Input: part model. Units: mm. Frame: model coordinates. A direction names the side the tool comes from. Coordinates: 2 decimals unless noted, no trailing zeros. Loops run counter-clockwise (first coordinate to the right, second up) from the corner with the lowest first, then second, coordinate; pieces in that order, holes last.
```python
from build123d import *

# Parameters (mm, degrees)
F2_DEPTH = 0.1
F3_ANGLE = 180
F4_ANGLE = 180
F5_DEPTH = 0.1
F6_R     = 0.2427611579
F7_DEPTH = 1


with BuildPart() as f2:
    # F1 (on Front) → F2 (new body)
    with BuildSketch(Plane.XZ):
        with BuildLine():
            Line((0, 0.6), (0, 0))
            Line((0, 0), (5, 0))
            Line((5, 0), (7.4486832981, 7.3460498942))
            ThreePointArc((7.4486832981, 7.3460498942), (7.4870874576, 7.5020954172), (7.5, 7.6622776602))
            Line((7.5, 7.6622776602), (7.5, 16.6690481052))
            ThreePointArc((7.5, 16.6690481052), (7.3911447846, 17.4698488508), (7.0724787771, 18.2125353714))
            Line((7.0724787771, 18.2125353714), (3.1456512734, 24.7572478777))
            ThreePointArc((3.1456512734, 24.7572478777), (2.963254218, 24.9350999534), (2.7169048105, 25))
            Line((2.7169048105, 25), (0, 25))
            Line((0, 25), (0, 24.4))
            Line((0, 24.4), (2.6383143499, 24.4))
            ThreePointArc((2.6383143499, 24.4), (2.6777302551, 24.3896159925), (2.7069137839, 24.3611596604))
            Line((2.7069137839, 24.3611596604), (6.5751328802, 17.9141278333))
            ThreePointArc((6.5751328802, 17.9141278333), (6.8321901263, 17.3150273733), (6.92, 16.6690481052))
            Line((6.92, 16.6690481052), (6.92, 7.6622776602))
            ThreePointArc((6.92, 7.6622776602), (6.9145767322, 7.5950011181), (6.8984469852, 7.5294619984))
            Line((6.8984469852, 7.5294619984), (4.588626319, 0.6))
            Line((4.588626319, 0.6), (0, 0.6))
        make_face()
    extrude(amount=F2_DEPTH)

    # F2_face (on face) → F3 (revolve)
    with BuildSketch(Plane(origin=(5.1843610202, -0.1, 11.965116571), x_dir=(1, 0, 0), z_dir=(0, -1, 0))):
        with BuildLine():
            Line((-0.5957347012, -11.365116571), (-5.1843610202, -11.365116571))
            Line((-5.1843610202, -11.365116571), (-5.1843610202, -11.965116571))
            Line((-5.1843610202, -11.965116571), (-0.1843610202, -11.965116571))
            Line((-0.1843610202, -11.965116571), (2.2643222778, -4.6190666769))
            ThreePointArc((2.2643222778, -4.6190666769), (2.3027264374, -4.4630211539), (2.3156389798, -4.3028389109))
            Line((2.3156389798, -4.3028389109), (2.3156389798, 4.7039315341))
            ThreePointArc((2.3156389798, 4.7039315341), (2.2067837644, 5.5047322798), (1.8881177569, 6.2474188004))
            Line((1.8881177569, 6.2474188004), (-2.0387097468, 12.7921313067))
            ThreePointArc((-2.0387097468, 12.7921313067), (-2.2211068022, 12.9699833824), (-2.4674562097, 13.034883429))
            Line((-2.4674562097, 13.034883429), (-5.1843610202, 13.034883429))
            Line((-5.1843610202, 13.034883429), (-5.1843610202, 12.434883429))
            Line((-5.1843610202, 12.434883429), (-2.5460466703, 12.434883429))
            ThreePointArc((-2.5460466703, 12.434883429), (-2.5066307651, 12.4244994215), (-2.4774472363, 12.3960430894))
            Line((-2.4774472363, 12.3960430894), (1.39077186, 5.9490112623))
            ThreePointArc((1.39077186, 5.9490112623), (1.6478291061, 5.3499108023), (1.7356389798, 4.7039315341))
            Line((1.7356389798, 4.7039315341), (1.7356389798, -4.3028389109))
            ThreePointArc((1.7356389798, -4.3028389109), (1.730215712, -4.3701154529), (1.714085965, -4.4356545726))
            Line((1.714085965, -4.4356545726), (-0.5957347012, -11.365116571))
        make_face()
    revolve(axis=Axis((0, -0.1, 24.7), (0, 0, -1)), revolution_arc=F3_ANGLE)

    # F1 (on Front) → F4 (revolve)
    with BuildSketch(Plane.XZ):
        with BuildLine():
            Line((0, 0.6), (0, 0))
            Line((0, 0), (5, 0))
            Line((5, 0), (7.4486832981, 7.3460498942))
            ThreePointArc((7.4486832981, 7.3460498942), (7.4870874576, 7.5020954172), (7.5, 7.6622776602))
            Line((7.5, 7.6622776602), (7.5, 16.6690481052))
            ThreePointArc((7.5, 16.6690481052), (7.3911447846, 17.4698488508), (7.0724787771, 18.2125353714))
            Line((7.0724787771, 18.2125353714), (3.1456512734, 24.7572478777))
            ThreePointArc((3.1456512734, 24.7572478777), (2.963254218, 24.9350999534), (2.7169048105, 25))
            Line((2.7169048105, 25), (0, 25))
            Line((0, 25), (0, 24.4))
            Line((0, 24.4), (2.6383143499, 24.4))
            ThreePointArc((2.6383143499, 24.4), (2.6777302551, 24.3896159925), (2.7069137839, 24.3611596604))
            Line((2.7069137839, 24.3611596604), (6.5751328802, 17.9141278333))
            ThreePointArc((6.5751328802, 17.9141278333), (6.8321901263, 17.3150273733), (6.92, 16.6690481052))
            Line((6.92, 16.6690481052), (6.92, 7.6622776602))
            ThreePointArc((6.92, 7.6622776602), (6.9145767322, 7.5950011181), (6.8984469852, 7.5294619984))
            Line((6.8984469852, 7.5294619984), (4.588626319, 0.6))
            Line((4.588626319, 0.6), (0, 0.6))
        make_face()
    revolve(axis=Axis((0, 0, 24.7), (0, 0, 1)), revolution_arc=F4_ANGLE)

    # F5 (add): a face of the model
    f5_faces = [f2.faces().sort_by_distance(p)[0] for p in [
        (-0.2610076627, -0.1, 0.3),
    ]]
    extrude(f5_faces, amount=F5_DEPTH)

    # F6 (on face) → F7 (cut)
    with BuildSketch(Plane(origin=(0, 0, 0), x_dir=(1, 0, 0), z_dir=(0, 0, -1))):
        Circle(F6_R)
    extrude(amount=-F7_DEPTH, mode=Mode.SUBTRACT)


solid = f2.part
```
Item 1: Section query A-A (z = 12.5). Output: boundary loops of the cut face in (x, y).
Result:
outline: (-7.5, -0.1) arc R7.5 ccw to (7.5, -0.1) - (7.5, 0) arc R7.5 ccw to (-7.5, 0) - close; hole (-6.92, -0.1) arc R6.92 ccw to (6.92, -0.1) - (6.92, 0) arc R6.92 ccw to (-6.92, 0) - close
Item 2: Reachability of faces 4 (the face through (0.15, -7.02, 12.1)), 5 (the face through (0.16, -7.6, 12.23)) from +Z, -Z, +X, -X, +Y, -Y: full face, straight path, thin tool, end or side. Return the list, or none.
Result:
face 4: none
face 5: +Z, -Z, -Y
Item 3: Line query: L1, parallel to Z at x = 2.5, y = -0.75; L2, parallel to X at y = 0, z = 0.4; L3, parallel to Z at x = -1.5, y = -4.25. Output: solid intervals per line, ascending.
Result:
L1: z = 0 to 0.6, 24.4 to 25
L2: x = -5.13 to -0.24, 0.24 to 5.13
L3: z = 0 to 0.6, 21.52 to 22.65
Item 4: Mould query, pull axis X, two halves, no side actions, for faces 1 (the face through (0.102, 4.644, 22.258)), 2 (the face through (0, 0, 25)), 3 (the face through (0.093, -4.337, 21.809)). Classes: +X half, -X half, draft (parallel to the pull), parting line (faces both ways), or undercut.
Result:
face 1: parting line
face 2: draft
face 3: undercut
Item 5: Contact query for flat-ended pins moving along their axis: P1, Ø1.5, axis at y = -0.5, z = 19.5, coming from the -X side; P2, Ø8, axis at y = -4.5, z = 15.5, coming from the +X side; P3, Ø1, axis at x = -5, y = -1.5, coming from the +Z side. Output: stop coordinate, or through.
Result:
P1: stops at x = -6.74
P2: stops at x = 7.49
P3: stops at z = 22.18
Item 6: Section query B-B (z = 3.75). Output: boundary loops of the cut face in (x, y), then the cut area to 3 significant figures.
Result:
outline: (-6.25, -0.1) arc R6.25 ccw to (6.25, -0.1) - (6.25, 0) arc R6.25 ccw to (-6.25, 0) - close; hole (-5.64, -0.1) arc R5.64 ccw to (5.64, -0.1) - (5.64, 0) arc R5.64 ccw to (-5.64, 0) - close
area: 23.0 mm2
